For this review, take the finished solid that the model builds, in its own axes (mm). Face numbers are marked on the shaded views. A direction names the side the tool comes from. Round coordinates to 2 decimals unless told otherwise and drop trailing zeros. Order: outer loops, then holes, each group sorted by start corner. A loop starts at its lowest first (then second) coordinate and runs counter-clockwise, first axis right, second up. Notation, with made-up numbers: (46, 10) - (105, 10) arc R30 cw to (105, 35) - close; hole circle Ø6 at (64, 47.25). An arc over 180 degrees is marked (long way). One line per question, with ' | ' between items.
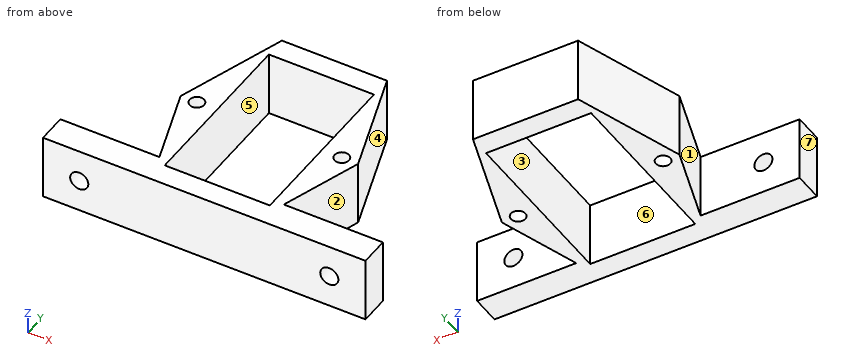
```python
from build123d import *

# Parameters (mm, degrees)
SKETCH_1_R          = 2
EXTRUDE_2_DEPTH     = 18
SKETCH_2_R          = 2.5
CUT_EXTRUDE_1_DEPTH = 18


with BuildPart() as part:
    # 草图1 → 凸台-拉伸2 (new body)
    with BuildSketch(Plane.XY):
        Polygon((2.302405498, 27.458762887), (-26.697594502, 27.458762887), (-36.697594502, -2.541237113), (-29.364261168, -24.541237113), (-56.697594502, -24.541237113), (-56.697594502, -32.541237113), (32.302405498, -32.541237113), (32.302405498, -24.541237113), (4.969072165, -24.541237113), (12.302405498, -2.541237113), align=None)
        with Locations((-32.197594502, -2.541237113)):
            Circle(SKETCH_1_R, mode=Mode.SUBTRACT)
        Polygon((-26.697594502, -26.541237113), (-26.697594502, -2.541237113), (-26.697594502, 21.458762887), (2.302405498, 21.458762887), (2.302405498, -2.541237113), (2.302405498, -26.541237113), align=None, mode=Mode.SUBTRACT)
        with Locations((7.802405498, -2.541237113)):
            Circle(SKETCH_1_R, mode=Mode.SUBTRACT)
    extrude(amount=EXTRUDE_2_DEPTH)

    # 草图2 → 切除-拉伸1 (cut)
    with BuildSketch(Plane(origin=(0, -24.541237113, 0), x_dir=(1, 0, 0), z_dir=(0, 1, 0))):
        with Locations(Location((-46.697594502, -9, 0), (0, 0, 270))):
            Circle(SKETCH_2_R)
        with Locations(Location((22.302405498, -9, 0), (0, 0, 270))):
            Circle(SKETCH_2_R)
    extrude(amount=-CUT_EXTRUDE_1_DEPTH, mode=Mode.SUBTRACT)


solid = part.part
```
(1) For the marked faces 1, 2 and 3, list the 3-axis set-ups (+Z, -Z, +X, -X, +Y, -Y) from which the entire face can be reached by the end or side of a thin tool; tool diameter is ignored.
Output values:
face 1: +Z, -Z, -X | face 2: +Z, -Z, +X | face 3: +Z, -Z
(2) We need section B-B on y = 13.5. State the section outline as (x, z) points, plus the area to 3 significant figures.
Output values:
outline: (-31.35, 0) - (-26.7, 0) - (-26.7, 18) - (-31.35, 18) - close; (2.3, 0) - (6.96, 0) - (6.96, 18) - (2.3, 18) - close | area: 168 mm^2
(3) We need section A-A on z = 9. State the section outline as (x, y) points.
Output values:
outline: (-56.7, -32.54) - (-49.2, -32.54) - (-49.2, -24.54) - (-56.7, -24.54) - close; (-44.2, -32.54) - (19.8, -32.54) - (19.8, -24.54) - (4.97, -24.54) - (12.3, -2.54) - (2.3, 27.46) - (-26.7, 27.46) - (-36.7, -2.54) - (-29.36, -24.54) - (-44.2, -24.54) - close; (24.8, -32.54) - (32.3, -32.54) - (32.3, -24.54) - (24.8, -24.54) - close; hole circle Ø4 at (-32.2, -2.54); hole (-26.7, -26.54) - (2.3, -26.54) - (2.3, 21.46) - (-26.7, 21.46) - close; hole circle Ø4 at (7.8, -2.54)
(4) Mouldability with a two-part tool opening along X and no side actions: class the marked faces 4, 5, 6 and 7 as released by +X, released by -X, zero draft, split by the parting line, or undercut.
Output values:
face 4: released by +X | face 5: undercut | face 6: undercut | face 7: released by -X
(5) For probe 1 along X at (y, z) = (-29, 9); probe 2 along X at (y, z) = (-26.5, 9); probe 3 along X at (y, z) = (19.5, 13), list the stretches that pass through material, from the lowest coordinate up. Write a range as [from, to].
Output values:
probe 1: [-56.7, -49.2], [-44.2, 19.8], [24.8, 32.3] | probe 2: [-56.7, -49.2], [-44.2, -26.7], [2.3, 19.8], [24.8, 32.3] | probe 3: [-29.35, -26.7], [2.3, 4.96]
(6) We need section C-C on y = -20. State the section outline as (x, z) points, plus the area to 3 significant figures.
Output values:
outline: (-30.88, 0) - (-26.7, 0) - (-26.7, 18) - (-30.88, 18) - close; (2.3, 0) - (6.48, 0) - (6.48, 18) - (2.3, 18) - close | area: 150 mm^2
(7) Insertion check: pin 1 (5 mm diameter, centred on y = -16.5, z = 3.5, fed in from +X); pin 2 (9 mm diameter, centred on y = -1.5, z = 10.5, fed in from -X); pin 3 (9 mm diameter, centred on x = -46.5, z = 6.5, fed in from +Y). Each pin has a flat end and moves straight along its axis. Give the tip position at first contact, or say it passes through.
Output values:
pin 1: x = 8.48 | pin 2: x = -36.7 | pin 3: y = -24.54
(8) We need section D-D on x = -39. State the section outline as (y, z) points.
Output values:
outline: (-32.54, 0) - (-24.54, 0) - (-24.54, 18) - (-32.54, 18) - close
